Model file for the job. Use its own axes, mm. Face numbers are marked on the shaded views. A direction names the side the tool comes from. Round coordinates to 2 decimals unless told otherwise and drop trailing zeros. Order: outer loops, then holes, each group sorted by start corner. A loop starts at its lowest first (then second) coordinate and runs counter-clockwise, first axis right, second up. Notation, with made-up numbers: (79, 22.25) - (113, 22.25) arc R34 cw to (113, 54.25) - close; hole circle Ø4 at (9, 61.5). An arc over 180 degrees is marked (long way). Write item = value, one per line.
```python
from build123d import *

# Parameters (mm, degrees)
ESBO_O1_W                = 70
ESBO_O1_H                = 27.14
RESSALTO_EXTRUS_O1_DEPTH = 5
ESBO_O2_R                = 1.5
CORTE_EXTRUS_O1_DEPTH    = 5
ESBO_O4_W                = 40.6
ESBO_O4_H                = 19.8
CORTE_EXTRUS_O2_DEPTH    = 6
ESBO_O5_R                = 1.5
CORTE_EXTRUS_O3_DEPTH    = 6


with BuildPart() as part:
    # Esboço1 → Ressalto-extrusão1 (new body)
    with BuildSketch(Plane.XY):
        with Locations((8.249487122, 6.106616915)):
            Rectangle(ESBO_O1_W, ESBO_O1_H)
    extrude(amount=RESSALTO_EXTRUS_O1_DEPTH)

    # Esboço2 → Corte-extrusão1 (cut)
    with BuildSketch(Plane.XY.offset(5)):
        with Locations((-24.250512878, 14.676616915)):
            Circle(ESBO_O2_R)
        with Locations((-24.250512878, -2.463383085)):
            Circle(ESBO_O2_R)
        with Locations((40.749487122, 11.106616915)):
            Circle(ESBO_O2_R)
        with Locations((40.749487122, 1.106616915)):
            Circle(ESBO_O2_R)
    extrude(amount=-CORTE_EXTRUS_O1_DEPTH, mode=Mode.SUBTRACT)

    # Esboço4 → Corte-extrusão2 (cut, through all)
    with BuildSketch(Plane(origin=(0, 0, 0), x_dir=(-1, 0, 0), z_dir=(0, 0, -1))):
        with Locations((-15.859487122, 6.106616915)):
            Rectangle(ESBO_O4_W, ESBO_O4_H)
    extrude(amount=-CORTE_EXTRUS_O2_DEPTH, mode=Mode.SUBTRACT)

    # Esboço5 → Corte-extrusão3 (cut, through all)
    with BuildSketch(Plane(origin=(0, 0, 0), x_dir=(-1, 0, 0), z_dir=(0, 0, -1))):
        with Locations((9.030512878, 1.106616915)):
            Circle(ESBO_O5_R)
        with Locations((9.030512878, 11.106616915)):
            Circle(ESBO_O5_R)
    extrude(amount=-CORTE_EXTRUS_O3_DEPTH, mode=Mode.SUBTRACT)


solid = part.part
```
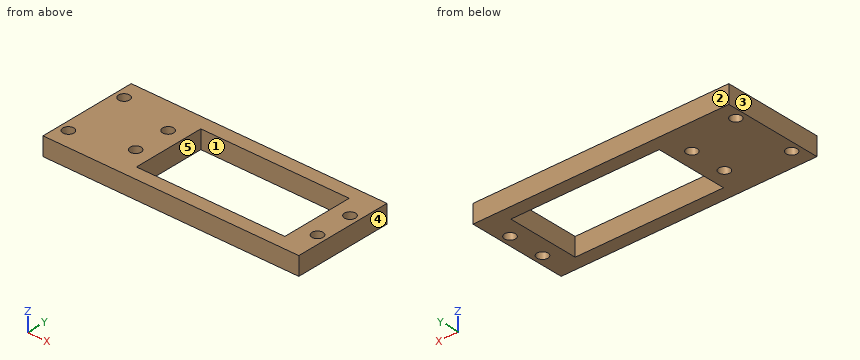
1) 3-axis set-ups, long thin cutter, end or side, ignore diameter. For the marked faces 4 and 5: which of +Z, -Z, +X, -X, +Y, -Y reach the whole face in a straight line?
Conclusion:
face_4 = +Z, -Z, +X, +Y, -Y
face_5 = +Z, -Z
2) Mould opens along X. For the marked faces 1, 2 and 3 say: +X half, -X half, draft (parallel to the pull), parting line (faces both ways), or undercut.
Conclusion:
face_1 = undercut
face_2 = draft
face_3 = -X half
3) Wall check: line 1 along X through (y, z) = (14.75, 4.75); line 2 along X through (y, z) = (9.5, 1.85); line 3 along Y through (x, z) = (3.5, 3.4). Give the ranges that are in metal, low to high.
Conclusion:
line_1 = -26.75 to -25.75, -22.75 to -4.44, 36.16 to 43.25
line_2 = -26.75 to -4.44, 36.16 to 43.25
line_3 = -7.46 to -3.79, 16.01 to 19.68
4) Cut at D-D (z = 4.1). Write the cut outline in (x, y).
Conclusion:
outline = (-26.75, -7.46) - (43.25, -7.46) - (43.25, 19.68) - (-26.75, 19.68) - close; hole circle Ø3 at (-24.25, -2.46); hole circle Ø3 at (-24.25, 14.68); hole circle Ø3 at (-9.03, 1.11); hole circle Ø3 at (-9.03, 11.11); hole (-4.44, -3.79) - (36.16, -3.79) - (36.16, 16.01) - (-4.44, 16.01) - close; hole circle Ø3 at (40.75, 1.11); hole circle Ø3 at (40.75, 11.11)
5) Cut at A-A (x = 2). Write the cut outline in (y, z), and give its area (3 significant figures).
Conclusion:
outline = (-7.46, 0) - (-3.79, 0) - (-3.79, 5) - (-7.46, 5) - close; (16.01, 0) - (19.68, 0) - (19.68, 5) - (16.01, 5) - close
area = 36.7 mm^2
6) Cut at B-B (y = 11.75). Write the cut outline in (x, z).
Conclusion:
outline = (-26.75, 0) - (-10.39, 0) - (-10.39, 5) - (-26.75, 5) - close; (-7.68, 0) - (-4.44, 0) - (-4.44, 5) - (-7.68, 5) - close; (36.16, 0) - (39.39, 0) - (39.39, 5) - (36.16, 5) - close; (42.1, 0) - (43.25, 0) - (43.25, 5) - (42.1, 5) - close
7) Cut at C-C (y = 7.25). Write the cut outline in (x, z), and give its area (3 significant figures).
Conclusion:
outline = (-26.75, 0) - (-4.44, 0) - (-4.44, 5) - (-26.75, 5) - close; (36.16, 0) - (43.25, 0) - (43.25, 5) - (36.16, 5) - close
area = 147 mm^2
